```python
from build123d import *

# Parameters (mm, degrees)
CROQUIS_BASE_R          = 10.982321859
SALIENTE_EXTRUIR1_DEPTH = 2.95
CROQUIS_BASE_3_R        = 1.568903123
CROQUIS_BASE_3_R_2      = 1.202825727
CORTAR_EXTRUIR1_DEPTH   = 2.95
CROQUIS_BASE_4_R        = 3.137806245
CORTAR_EXTRUIR2_DEPTH   = 1.05
CROQUIS2_R              = 4.4
SALIENTE_EXTRUIR2_DEPTH = 2.7
CROQUIS3_R              = 3
CORTAR_EXTRUIR3_DEPTH   = 3.5


with BuildPart() as part:
    # Croquis base → Saliente-Extruir1 (new body)
    with BuildSketch(Plane(origin=(0, 0, 0), x_dir=(1, 0, 0), z_dir=(0, 1, 0))):
        with Locations(Location((0, 0, 0), (0, 0, 270))):
            Circle(CROQUIS_BASE_R)
    extrude(amount=SALIENTE_EXTRUIR1_DEPTH)

    # Croquis base_3 → Cortar-Extruir1 (cut)
    with BuildSketch(Plane(origin=(0, 0, 0), x_dir=(1, 0, 0), z_dir=(0, 1, 0))):
        with Locations(Location((0, 0, 0), (0, 0, 270))):
            Circle(CROQUIS_BASE_3_R)
        with Locations(Location((-7.35, 0, 0), (0, 0, 270))):
            Circle(CROQUIS_BASE_3_R_2)
        with Locations(Location((0, 7.35, 0), (0, 0, 270))):
            Circle(CROQUIS_BASE_3_R_2)
        with Locations(Location((7.35, 0, 0), (0, 0, 270))):
            Circle(CROQUIS_BASE_3_R_2)
        with Locations(Location((0, -7.35, 0), (0, 0, 270))):
            Circle(CROQUIS_BASE_3_R_2)
    extrude(amount=CORTAR_EXTRUIR1_DEPTH, mode=Mode.SUBTRACT)

    # Croquis base_4 → Cortar-Extruir2 (cut)
    with BuildSketch(Plane(origin=(0, 0, 0), x_dir=(1, 0, 0), z_dir=(0, 1, 0))):
        with Locations(Location((0, 0, 0), (0, 0, 270))):
            Circle(CROQUIS_BASE_4_R)
    extrude(amount=CORTAR_EXTRUIR2_DEPTH, mode=Mode.SUBTRACT)

    # Croquis2 → Saliente-Extruir2 (add)
    with BuildSketch(Plane(origin=(0, 2.95, 0), x_dir=(1, 0, 0), z_dir=(0, 1, 0))):
        with Locations(Location((0, 0, 0), (0, 0, 90))):
            Circle(CROQUIS2_R)
    extrude(amount=SALIENTE_EXTRUIR2_DEPTH)

    # Croquis3 → Cortar-Extruir3 (cut)
    with BuildSketch(Plane(origin=(0, 5.65, 0), x_dir=(1, 0, 0), z_dir=(0, 1, 0))):
        with Locations(Location((0, 0, 0), (0, 0, 270))):
            Circle(CROQUIS3_R)
    extrude(amount=-CORTAR_EXTRUIR3_DEPTH, mode=Mode.SUBTRACT)


solid = part.part
```
Geometry: final body of the model. Coordinates: model frame, mm. A direction names the side the tool comes from. Round coordinates to 2 decimals unless told otherwise and drop trailing zeros. Write each loop counter-clockwise with the first axis right and the second up, starting at its lowest first coordinate (ties: lowest second). Pieces come first, ordered by that corner, then holes. Notation, with made-up numbers: (-9.5, -35.5) -> (19.5, -35.5) arc R9 ccw to (19.5, -20.5) -> close; hole circle Ø10 at (-25, -14). An arc over 180 degrees is marked (long way). Return JSON: item names as keys, results as strings.
Q1. Mould query, pull axis Z, two halves, no side actions, for faces 1 (the flat face through (0, 2.95, 5)), 2 (the cylindrical face through (6.176, 1.454, -0.261)), 3 (the cylindrical face through (-6.7, 1.5, -8.7)). Classes: +Z half, -Z half, draft (parallel to the pull), parting line (faces both ways), or undercut.
From the geometry:
{"face 1": "draft", "face 2": "undercut", "face 3": "parting line"}
Q2. First-contact query: pin 1 Ø4 at (x, z) = (0, 7.35) entering from -Y; pin 2 Ø1.4 at (x, z) = (0, -7.35) entering from -Y; pin 3 Ø2 at (y, z) = (3.5, 6.5) entering from +X; pin 4 Ø1 at (x, z) = (8.5, -7.5) entering from +Y. Flat tips, straight axial feed; report the tip coordinate or a pass-through.
From the geometry:
{"pin 1": "y = 0", "pin 2": "through", "pin 3": "x = 9.41", "pin 4": "y = 2.95"}
Q3. Ray query, line 1 (X direction, y = 1.8, z = 0); line 2 (Y direction, x = -5, z = -9.5); line 3 (Z direction, x = 2.5, y = 3.9). Return the intervals inside material, ascending.
From the geometry:
{"line 1": "-10.98 to -8.55, -6.15 to -1.57, 1.57 to 6.15, 8.55 to 10.98", "line 2": "0 to 2.95", "line 3": "-3.62 to -1.66, 1.66 to 3.62"}
Q4. Set-up query: faces 4 (the cylindrical face through (0.9, 3.92, 2.86)), 5 (the cylindrical face through (0.05, 1.45, -8.55)), 6 (the flat face through (-1.4, 1.05, 1.4)). Return all of +Z, -Z, +X, -X, +Y, -Y with unobstructed straight access to the full face (end or side cutting, diameter ignored); none if empty.
From the geometry:
{"face 4": "+Y", "face 5": "+Y, -Y", "face 6": "-Y"}
Q5. Section D-D on x = -7. Return the cut outline in (y, z).
From the geometry:
{"outline": "(0, -8.46) -> (2.95, -8.46) -> (2.95, -1.15) -> (0, -1.15) -> close; (0, 1.15) -> (2.95, 1.15) -> (2.95, 8.46) -> (0, 8.46) -> close"}
Q6. Section A-A on z = 0. Return the cut outline in (x, y), and give its area (3 significant figures).
From the geometry:
{"outline": "(-10.98, 0) -> (-8.55, 0) -> (-8.55, 2.95) -> (-10.98, 2.95) -> close; (-6.15, 0) -> (-3.14, 0) -> (-3.14, 1.05) -> (-1.57, 1.05) -> (-1.57, 2.15) -> (-3, 2.15) -> (-3, 5.65) -> (-4.4, 5.65) -> (-4.4, 2.95) -> (-6.15, 2.95) -> close; (1.57, 1.05) -> (3.14, 1.05) -> (3.14, 0) -> (6.15, 0) -> (6.15, 2.95) -> (4.4, 2.95) -> (4.4, 5.65) -> (3, 5.65) -> (3, 2.15) -> (1.57, 2.15) -> close; (8.55, 0) -> (10.98, 0) -> (10.98, 2.95) -> (8.55, 2.95) -> close", "area": "43.3 mm2"}
Q7. Section B-B on x = 0. Return the cut outline in (y, z), and give its area (3 significant figures).
From the geometry:
{"outline": "(0, -10.98) -> (2.95, -10.98) -> (2.95, -8.55) -> (0, -8.55) -> close; (0, -6.15) -> (2.95, -6.15) -> (2.95, -4.4) -> (5.65, -4.4) -> (5.65, -3) -> (2.15, -3) -> (2.15, -1.57) -> (1.05, -1.57) -> (1.05, -3.14) -> (0, -3.14) -> close; (0, 3.14) -> (1.05, 3.14) -> (1.05, 1.57) -> (2.15, 1.57) -> (2.15, 3) -> (5.65, 3) -> (5.65, 4.4) -> (2.95, 4.4) -> (2.95, 6.15) -> (0, 6.15) -> close; (0, 8.55) -> (2.95, 8.55) -> (2.95, 10.98) -> (0, 10.98) -> close", "area": "43.3 mm2"}
Q8. Section C-C on y = 4.85. Return the cut outline in (x, z), and give its area (3 significant figures).
From the geometry:
{"outline": "circle Ø8.8 at (0, 0); hole circle Ø6 at (0, 0)", "area": "32.5 mm2"}
